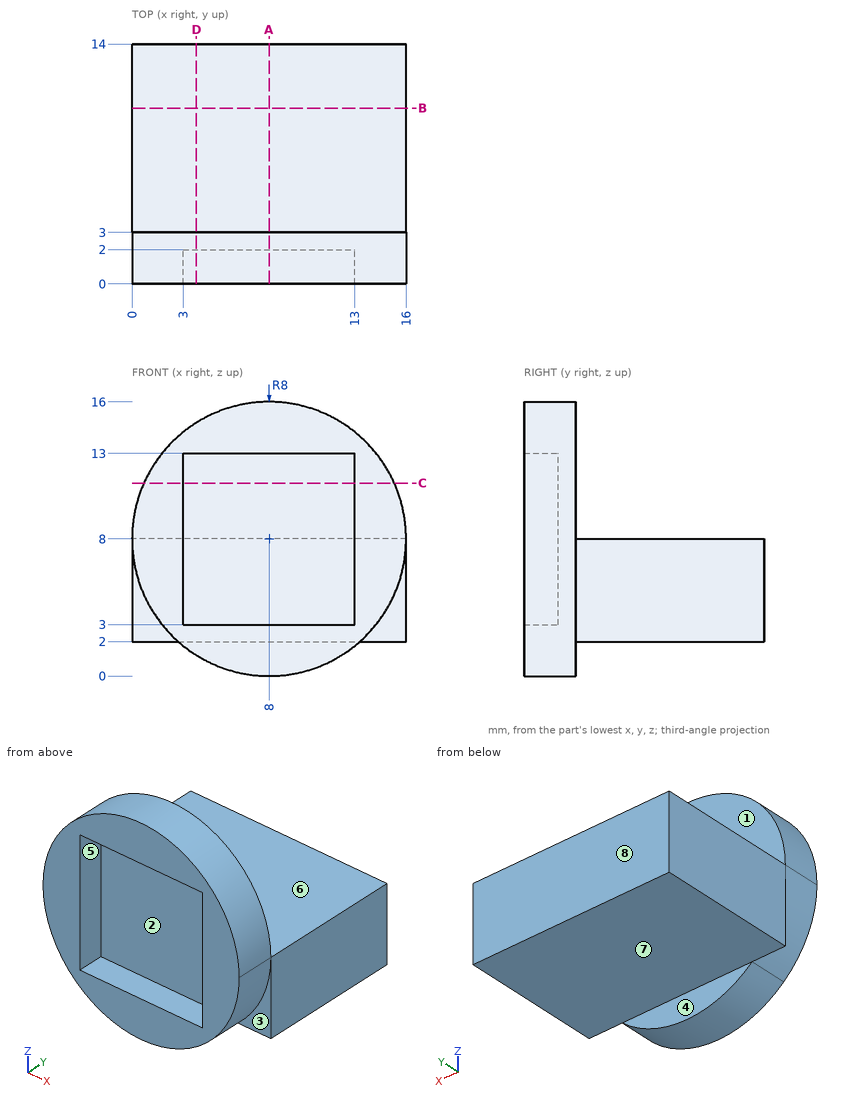
Geometry: see drawing. Coordinates: mm, zero at the bounding-box minimum. A direction names the side the tool comes from. Give positions to 0.01 mm unless a question says otherwise; leave off trailing zeros. Order: outer loops, then holes, each group sorted by start corner. A loop starts at its lowest first (then second) coordinate and runs counter-clockwise, first axis right, second up. Notation, with made-up numbers: (57.5, -4) -> (63.5, -4) arc R27 ccw to (63.5, 20) -> close; hole circle Ø10 at (37.5, 6.25). An arc over 180 degrees is marked (long way). Write each question's results on one line, items separated by ' | '.
1) Line query: line 1 along Z through (x, y) = (1.25, 5.25); line 2 along Y through (x, z) = (3.75, 12); line 3 along Y through (x, z) = (6, 15). Output: solid intervals per line, ascending.
Geometry says:
line 1: z = 2 to 8 | line 2: y = 2 to 3 | line 3: y = 0 to 3
2) Draft query along Z for the marked faces 5, 6, 7 and 8. Return one class per face: released by +Z, released by -Z, zero draft, split by the parting line, or undercut.
Geometry says:
face 5: undercut | face 6: released by +Z | face 7: released by -Z | face 8: zero draft
3) Cut plane A-A (x = 8). Output: boundary loops of the cut face in (y, z), and give its area (3 significant figures).
Geometry says:
outline: (0, 0) -> (3, 0) -> (3, 2) -> (14, 2) -> (14, 8) -> (3, 8) -> (3, 16) -> (0, 16) -> (0, 13) -> (2, 13) -> (2, 3) -> (0, 3) -> close | area: 94.0 mm²
4) Cut plane C-C (z = 11.25). Output: boundary loops of the cut face in (x, y).
Geometry says:
outline: (0.69, 0) -> (3, 0) -> (3, 2) -> (13, 2) -> (13, 0) -> (15.31, 0) -> (15.31, 3) -> (0.69, 3) -> close
5) First-contact query: pin 1 Ø2.5 at (x, z) = (7.5, 11) entering from +Y; pin 2 Ø4 at (y, z) = (4, 11.5) entering from -X; pin 3 Ø8 at (x, y) = (5, 8) entering from -Z. Flat tips, straight axial feed; report the tip coordinate or a pass-through.
Geometry says:
pin 1: stops at y = 3 | pin 2: stops at x = 0.2 | pin 3: stops at z = 2
6) Set-up query: the marked faces 1, 2, 3 and 4. Return all of +Z, -Z, +X, -X, +Y, -Y with unobstructed straight access to the full face (end or side cutting, diameter ignored); none if empty.
Geometry says:
face 1: +Z, +X, -X, +Y | face 2: -Y | face 3: -Z, +X, -Y | face 4: -Z, +X, -X, +Y
7) Cut plane D-D (x = 3.75). Output: boundary loops of the cut face in (y, z).
Geometry says:
outline: (0, 1.22) -> (3, 1.22) -> (3, 2) -> (14, 2) -> (14, 8) -> (3, 8) -> (3, 14.78) -> (0, 14.78) -> (0, 13) -> (2, 13) -> (2, 3) -> (0, 3) -> close
8) Cut plane B-B (y = 10.25). Output: boundary loops of the cut face in (x, z), and give its area (3 significant figures).
Geometry says:
outline: (0, 2) -> (16, 2) -> (16, 8) -> (0, 8) -> close | area: 96.0 mm²
